Geometry: final body of the model. Coordinates: model frame, mm. Give positions to 0.01 mm unless a question says otherwise; leave off trailing zeros. Answer as a JSON object with one key per item and string values. Group by question number.
(1) Section query A-A on z = -40. State how many separate pieces and enclosed holes the cut face has, plus the area to 3 significant figures.
(2) Contact query for flat-ended pins moving along their axis: pin 1 Ø6 at (y, z) = (-1.5, -91) entering from -X; pin 2 Ø1.2 at (x, z) = (-2, -249) entering from -Y. Output: stop coordinate, or through.
(3) Material intervals for probe 1 along Y at (x, z) = (-3.68, -120); probe 2 along Y at (x, z) = (-3.75, -40.5); probe 3 along X at (y, z) = (4, -30), sorted ascending.
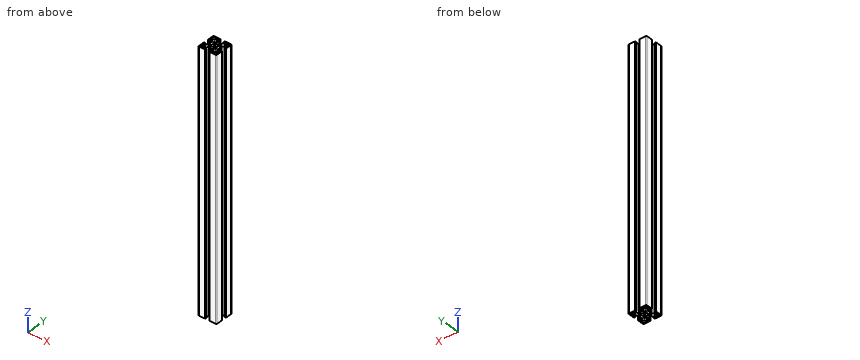
from build123d import *

# Parameters (mm, degrees)
BOSS_EXTRUDE1_DEPTH = 350


with BuildPart() as part:
    # Sketch1 → Boss-Extrude1 (new body)
    with BuildSketch(Plane(origin=(0, 0, -350), x_dir=(-1, 0, 0), z_dir=(0, 0, -1))):
        with BuildLine():
            Line((12.5, -3), (10.5, -3))
            Line((10.5, -3), (10.5, -6))
            Line((10.5, -6), (9.535533906, -6))
            Line((9.535533906, -6), (6.5, -2.964466094))
            Line((6.5, -2.964466094), (6.5, -0.519615242))
            Line((6.5, -0.519615242), (6.2, 0))
            Line((6.2, 0), (6.5, 0.519615242))
            Line((6.5, 0.519615242), (6.5, 2.964466094))
            Line((6.5, 2.964466094), (9.535533906, 6))
            Line((9.535533906, 6), (10.5, 6))
            Line((10.5, 6), (10.5, 3))
            Line((10.5, 3), (12.5, 3))
            Line((12.5, 3), (12.5, 11.5))
            ThreePointArc((12.5, 11.5), (12.207106781, 12.207106781), (11.5, 12.5))
            Line((11.5, 12.5), (3, 12.5))
            Line((3, 12.5), (3, 10.5))
            Line((3, 10.5), (6, 10.5))
            Line((6, 10.5), (6, 9.535533906))
            Line((6, 9.535533906), (2.964466094, 6.5))
            Line((2.964466094, 6.5), (0.519615242, 6.5))
            Line((0.519615242, 6.5), (0, 6.2))
            Line((0, 6.2), (-0.519615242, 6.5))
            Line((-0.519615242, 6.5), (-2.964466094, 6.5))
            Line((-2.964466094, 6.5), (-6, 9.535533906))
            Line((-6, 9.535533906), (-6, 10.5))
            Line((-6, 10.5), (-3, 10.5))
            Line((-3, 10.5), (-3, 12.5))
            Line((-3, 12.5), (-11.5, 12.5))
            ThreePointArc((-11.5, 12.5), (-12.207106781, 12.207106781), (-12.5, 11.5))
            Line((-12.5, 11.5), (-12.5, 3))
            Line((-12.5, 3), (-10.5, 3))
            Line((-10.5, 3), (-10.5, 6))
            Line((-10.5, 6), (-9.535533906, 6))
            Line((-9.535533906, 6), (-6.5, 2.964466094))
            Line((-6.5, 2.964466094), (-6.5, 0.519615242))
            Line((-6.5, 0.519615242), (-6.2, 0))
            Line((-6.2, 0), (-6.5, -0.519615242))
            Line((-6.5, -0.519615242), (-6.5, -2.964466094))
            Line((-6.5, -2.964466094), (-9.535533906, -6))
            Line((-9.535533906, -6), (-10.5, -6))
            Line((-10.5, -6), (-10.5, -3))
            Line((-10.5, -3), (-12.5, -3))
            Line((-12.5, -3), (-12.5, -11.5))
            ThreePointArc((-12.5, -11.5), (-12.207106781, -12.207106781), (-11.5, -12.5))
            Line((-11.5, -12.5), (-3, -12.5))
            Line((-3, -12.5), (-3, -10.5))
            Line((-3, -10.5), (-6, -10.5))
            Line((-6, -10.5), (-6, -9.535533906))
            Line((-6, -9.535533906), (-2.964466094, -6.5))
            Line((-2.964466094, -6.5), (-0.519615242, -6.5))
            Line((-0.519615242, -6.5), (0, -6.2))
            Line((0, -6.2), (0.519615242, -6.5))
            Line((0.519615242, -6.5), (2.964466094, -6.5))
            Line((2.964466094, -6.5), (6, -9.535533906))
            Line((6, -9.535533906), (6, -10.5))
            Line((6, -10.5), (3, -10.5))
            Line((3, -10.5), (3, -12.5))
            Line((3, -12.5), (11.5, -12.5))
            ThreePointArc((11.5, -12.5), (12.207106781, -12.207106781), (12.5, -11.5))
            Line((12.5, -11.5), (12.5, -3))
        make_face()
        with BuildLine():
            Line((3.087755464, -1.885673936), (3.585519377, -2.383437849))
            ThreePointArc((3.585519377, -2.383437849), (4.599238816, -4.599238816), (2.383437849, -3.585519377))
            Line((2.383437849, -3.585519377), (1.885673936, -3.087755464))
            ThreePointArc((1.885673936, -3.087755464), (1.720751743, -3.0036254), (1.537849315, -3.032329053))
            ThreePointArc((1.537849315, -3.032329053), (0, -3.4), (-1.537849315, -3.032329053))
            ThreePointArc((-1.537849315, -3.032329053), (-1.720751743, -3.0036254), (-1.885673936, -3.087755464))
            Line((-1.885673936, -3.087755464), (-2.383437849, -3.585519377))
            ThreePointArc((-2.383437849, -3.585519377), (-4.599238816, -4.599238816), (-3.585519377, -2.383437849))
            Line((-3.585519377, -2.383437849), (-3.087755464, -1.885673936))
            ThreePointArc((-3.087755464, -1.885673936), (-3.0036254, -1.720751743), (-3.032329053, -1.537849315))
            ThreePointArc((-3.032329053, -1.537849315), (-3.4, 0), (-3.032329053, 1.537849315))
            ThreePointArc((-3.032329053, 1.537849315), (-3.0036254, 1.720751743), (-3.087755464, 1.885673936))
            Line((-3.087755464, 1.885673936), (-3.585519377, 2.383437849))
            ThreePointArc((-3.585519377, 2.383437849), (-4.599238816, 4.599238816), (-2.383437849, 3.585519377))
            Line((-2.383437849, 3.585519377), (-1.885673936, 3.087755464))
            ThreePointArc((-1.885673936, 3.087755464), (-1.720751743, 3.0036254), (-1.537849315, 3.032329053))
            ThreePointArc((-1.537849315, 3.032329053), (0, 3.4), (1.537849315, 3.032329053))
            ThreePointArc((1.537849315, 3.032329053), (1.720751743, 3.0036254), (1.885673936, 3.087755464))
            Line((1.885673936, 3.087755464), (2.383437849, 3.585519377))
            ThreePointArc((2.383437849, 3.585519377), (4.599238816, 4.599238816), (3.585519377, 2.383437849))
            Line((3.585519377, 2.383437849), (3.087755464, 1.885673936))
            ThreePointArc((3.087755464, 1.885673936), (3.0036254, 1.720751743), (3.032329053, 1.537849315))
            ThreePointArc((3.032329053, 1.537849315), (3.4, 0), (3.032329053, -1.537849315))
            ThreePointArc((3.032329053, -1.537849315), (3.0036254, -1.720751743), (3.087755464, -1.885673936))
        make_face(mode=Mode.SUBTRACT)
        with BuildLine():
            Line((11.25, -7.976197667), (11.25, -9.75))
            ThreePointArc((11.25, -9.75), (10.810660172, -10.810660172), (9.75, -11.25))
            Line((9.75, -11.25), (7.976197667, -11.25))
            ThreePointArc((7.976197667, -11.25), (7.329481994, -10.817878403), (7.48122292, -10.055025253))
            Line((7.48122292, -10.055025253), (8.061017306, -9.475230868))
            Line((8.061017306, -9.475230868), (7.353910524, -8.768124087))
            ThreePointArc((7.353910524, -8.768124087), (7.353910524, -7.353910524), (8.768124087, -7.353910524))
            Line((8.768124087, -7.353910524), (9.475230868, -8.061017306))
            Line((9.475230868, -8.061017306), (10.055025253, -7.48122292))
            ThreePointArc((10.055025253, -7.48122292), (10.817878403, -7.329481994), (11.25, -7.976197667))
        make_face(mode=Mode.SUBTRACT)
        with BuildLine():
            Line((-8.061017306, 9.475230868), (-7.353910524, 8.768124087))
            ThreePointArc((-7.353910524, 8.768124087), (-7.353910524, 7.353910524), (-8.768124087, 7.353910524))
            Line((-8.768124087, 7.353910524), (-9.475230868, 8.061017306))
            Line((-9.475230868, 8.061017306), (-10.055025253, 7.48122292))
            ThreePointArc((-10.055025253, 7.48122292), (-10.817878403, 7.329481994), (-11.25, 7.976197667))
            Line((-11.25, 7.976197667), (-11.25, 9.75))
            ThreePointArc((-11.25, 9.75), (-10.810660172, 10.810660172), (-9.75, 11.25))
            Line((-9.75, 11.25), (-7.976197667, 11.25))
            ThreePointArc((-7.976197667, 11.25), (-7.329481994, 10.817878403), (-7.48122292, 10.055025253))
            Line((-7.48122292, 10.055025253), (-8.061017306, 9.475230868))
        make_face(mode=Mode.SUBTRACT)
        with BuildLine():
            Line((-9.475230868, -8.061017306), (-8.768124087, -7.353910524))
            ThreePointArc((-8.768124087, -7.353910524), (-7.353910524, -7.353910524), (-7.353910524, -8.768124087))
            Line((-7.353910524, -8.768124087), (-8.061017306, -9.475230868))
            Line((-8.061017306, -9.475230868), (-7.48122292, -10.055025253))
            ThreePointArc((-7.48122292, -10.055025253), (-7.329481994, -10.817878403), (-7.976197667, -11.25))
            Line((-7.976197667, -11.25), (-9.75, -11.25))
            ThreePointArc((-9.75, -11.25), (-10.810660172, -10.810660172), (-11.25, -9.75))
            Line((-11.25, -9.75), (-11.25, -7.976197667))
            ThreePointArc((-11.25, -7.976197667), (-10.817878403, -7.329481994), (-10.055025253, -7.48122292))
            Line((-10.055025253, -7.48122292), (-9.475230868, -8.061017306))
        make_face(mode=Mode.SUBTRACT)
        with BuildLine():
            Line((11.25, 9.75), (11.25, 7.976197667))
            ThreePointArc((11.25, 7.976197667), (10.817878403, 7.329481994), (10.055025253, 7.48122292))
            Line((10.055025253, 7.48122292), (9.475230868, 8.061017306))
            Line((9.475230868, 8.061017306), (8.768124087, 7.353910524))
            ThreePointArc((8.768124087, 7.353910524), (7.353910524, 7.353910524), (7.353910524, 8.768124087))
            Line((7.353910524, 8.768124087), (8.061017306, 9.475230868))
            Line((8.061017306, 9.475230868), (7.48122292, 10.055025253))
            ThreePointArc((7.48122292, 10.055025253), (7.329481994, 10.817878403), (7.976197667, 11.25))
            Line((7.976197667, 11.25), (9.75, 11.25))
            ThreePointArc((9.75, 11.25), (10.810660172, 10.810660172), (11.25, 9.75))
        make_face(mode=Mode.SUBTRACT)
    extrude(amount=-BOSS_EXTRUDE1_DEPTH)


solid = part.part
Answer list:
{
 "1": {"separate pieces": "1", "enclosed holes": "5", "area": "302 mm2"},
 "2": {"pin 1": "x = -12.5", "pin 2": "y = -6.5"},
 "3": {"probe 1": "-12.5 to -10.5, -7.22 to -4.98, -2.38 to 2.38, 4.98 to 7.22, 10.5 to 12.5", "probe 2": "-12.5 to -10.5, -7.29 to -4.98, -2.38 to 2.38, 4.98 to 7.29, 10.5 to 12.5", "probe 3": "-12.5 to -10.5, -7.54 to -4.94, -2.42 to 2.42, 4.94 to 7.54, 10.5 to 12.5"}
}
